Model file for the job. Use its own axes, mm. A direction names the side the tool comes from. Coordinates: 2 decimals unless noted, no trailing zeros. Loops run counter-clockwise (first coordinate to the right, second up) from the corner with the lowest first, then second, coordinate; pieces in that order, holes last. Notation, with made-up numbers: (37.5, 14.5) - (75.5, 14.5) arc R9 ccw to (75.5, 20.5) - close; hole circle Ø9 at (-36.5, -40). An arc over 180 degrees is marked (long way). Write each question's results on one line, items separated by ' | '. Start each with the question number.
```python
from build123d import *

# Parameters (mm, degrees)
F0_W     = 10
F0_H     = 1.2
F1_DEPTH = 30
F2_W     = 10
F2_H     = 4
F2_R     = 1.25
F3_DEPTH = 47.801
F4_DEPTH = 2.4
F5_R     = 5
F6_DEPTH = 25
F7_R     = 2
F7_R_2   = 6.75
F8_DEPTH = 3


# Not quite as in the source:
# - a feature names something its author has since deleted; it is built from what else it names


with BuildPart() as f1:
    # F0 (on Top) → F1 (new body)
    with BuildSketch(Plane.XY):
        with BuildLine():
            Line((15, -11.6619037897), (15, -21.5))
            Line((15, -21.5), (5, -21.5))
            Line((5, -21.5), (5, -22.7))
            Line((5, -22.7), (5, -23.9))
            Line((5, -23.9), (17.4, -23.9))
            Line((17.4, -23.9), (17.4, -13.462540622))
            ThreePointArc((17.4, -13.462540622), (22, 0), (17.4, 13.462540622))
            Line((17.4, 13.462540622), (17.4, 23.9))
            Line((17.4, 23.9), (5, 23.9))
            Line((5, 23.9), (5, 22.7))
            Line((5, 22.7), (5, 21.5))
            Line((5, 21.5), (15, 21.5))
            Line((15, 21.5), (15, 11.6619037897))
            ThreePointArc((15, 11.6619037897), (19, 0), (15, -11.6619037897))
        make_face()
        with Locations((0, 23.3)):
            Rectangle(F0_W, F0_H)
        with BuildLine():
            Line((-5, -23.9), (-5, -22.7))
            Line((-5, -22.7), (-5, -21.5))
            Line((-5, -21.5), (-15, -21.5))
            Line((-15, -21.5), (-15, -11.6619037897))
            ThreePointArc((-15, -11.6619037897), (-19, 0), (-15, 11.6619037897))
            Line((-15, 11.6619037897), (-15, 21.5))
            Line((-15, 21.5), (-5, 21.5))
            Line((-5, 21.5), (-5, 22.7))
            Line((-5, 22.7), (-5, 23.9))
            Line((-5, 23.9), (-17.4, 23.9))
            Line((-17.4, 23.9), (-17.4, 13.462540622))
            ThreePointArc((-17.4, 13.462540622), (-22, 0), (-17.4, -13.462540622))
            Line((-17.4, -13.462540622), (-17.4, -23.9))
            Line((-17.4, -23.9), (-5, -23.9))
        make_face()
        with Locations((0, -23.3)):
            Rectangle(F0_W, F0_H)
    extrude(amount=F1_DEPTH)

    # F2 (on face) → F3 (cut, through all)
    with BuildSketch(Plane.XZ.offset(23.9)):
        with Locations((0, 22)):
            Rectangle(F2_W, F2_H)
        with Locations((0, 8)):
            Rectangle(F2_W, F2_H)
        with Locations((0, 15)):
            Circle(F2_R)
    extrude(amount=-F3_DEPTH, mode=Mode.SUBTRACT)

    # F0 (on Top) → F4 (cut)
    with BuildSketch(Plane.XY):
        with Locations((0, 23.3)):
            Rectangle(F0_W, F0_H)
        with Locations((0, -23.3)):
            Rectangle(F0_W, F0_H)
    extrude(amount=F4_DEPTH, mode=Mode.SUBTRACT)

    # F5
    f5_edges = [f1.edges().sort_by_distance(p)[0] for p in [
        (-17.4, -23.9, 15),
        (17.4, -23.9, 15),
        (-17.4, -13.462541, 15),
        (-17.4, 23.9, 15),
        (17.4, 23.9, 15),
        (17.4, -13.462541, 15),
    ]]
    fillet(f5_edges, radius=F5_R)

    # F6 (add): a face of the model
    f6_faces = [f1.faces().sort_by_distance(p)[0] for p in [
        (16.7503200788, -16.9872408745, 30),
    ]]
    extrude(f6_faces, amount=F6_DEPTH)

    # F7 (on face) → F8 (join)
    with BuildSketch(Plane.XY.offset(55)):
        Polygon((-15, -11.6619037897), (-15, -21.5), (-5, -21.5), (5, -21.5), (15, -21.5), (15, -11.6619037897), (15, 11.6619037897), (15, 21.5), (5, 21.5), (-5, 21.5), (-15, 21.5), (-15, 11.6619037897), align=None)
        with Locations((0, -12.5)):
            Circle(F7_R, mode=Mode.SUBTRACT)
        Circle(F7_R_2, mode=Mode.SUBTRACT)
        with Locations((0, 12.5)):
            Circle(F7_R, mode=Mode.SUBTRACT)
    extrude(amount=-F8_DEPTH)


solid = f1.part
```
Q1. Cut at D-D (x = -9). List the corners of the cut face in (y, z).
Q2. Mould opens along X. For faces 1 (the flat face through (-10, 21.5, 26)), 2 (the flat face through (0, 22.7, 39)), 3 (the flat face through (-19.2, 0.1, 0)), 4 (the flat face through (17.4, 16, 27)) say: +X half, -X half, draft (parallel to the pull), parting line (faces both ways), or undercut.
Q3. Which spindle directions (+Z, -Z, +X, -X, +Y, -Y) get a long thin tool onto all of the face, cutting with end or side? Do faces 5 (the flat face through (10, 21.5, 26)), 6 (the flat face through (17.4, -17, 27)), 7 (the flat face through (-1, -22.7, 16)). Say none if no direction does.
Q4. Drill centre lines: L1, parallel to Z at x = 0, y = 23.3; L2, parallel to Y at x = 0, z = 53.5; L3, parallel to X at y = 17.5, z = 46.5. Where is each one in solid material? Low to high. Write a range as from..to.
Q5. Pin check, flat tips, straight feed: pin 1 (15 mm diameter, centred on x = 5.5, y = 2, fed in from -Z); pin 2 (8 mm diameter, centred on x = 15.5, y = -17.5, fed in from -Z); pin 3 (3 mm diameter, centred on y = 7, z = 15, fed in from -X); pin 4 (10 mm diameter, centred on y = 8.5, z = 23.5, fed in from -X). Stop position of each tip, or through.
Q6. Cut at A-A (y = 0). List the corners of the cut face in (x, z), and give its area (4 significant figures).
Check result:
1) outline: (-23.9, 0) - (-21.5, 0) - (-21.5, 52) - (21.5, 52) - (21.5, 0) - (23.9, 0) - (23.9, 55) - (-23.9, 55) - close
2) face 1: undercut | face 2: undercut | face 3: draft | face 4: +X half
3) face 5: -Z | face 6: +Z, -Z, +X, -Y | face 7: +Z, -Z
4) L1: 2.4..6, 10..13.75, 16.25..20, 24..55 | L2: -23.9..-22.7, -21.5..-14.5, -10.5..-6.75, 6.75..10.5, 14.5..21.5, 22.7..23.9 | L3: -17.4..-15, 15..17.4
5) pin 1: z = 52 | pin 2: z = 0 | pin 3: x = -21.3 | pin 4: x = -21.72
6) outline: (-22, 0) - (-19, 0) - (-19, 55) - (-22, 55) - close; (-15, 52) - (-6.75, 52) - (-6.75, 55) - (-15, 55) - close; (6.75, 52) - (15, 52) - (15, 55) - (6.75, 55) - close; (19, 0) - (22, 0) - (22, 55) - (19, 55) - close | area: 379.5 mm²
